Can you work these out from the drawing? Everything is in mm from the part's minimum corner. Coordinates: 2 decimals unless noted, no trailing zeros. Order: outer loops, then holes, each group sorted by start corner. A loop starts at its lowest first (then second) coordinate and runs counter-clockwise, first axis right, second up. Notation, with made-up numbers: (-23, 41) -> (-8, 41) arc R29 cw to (-8, 66) -> close; hole circle Ø7 at (61, -15). An arc over 180 degrees is marked (long way). Use a Markdown table: item, result. Add a question column.
1) Will these pins go through, and if not, where does the flat tip stop? pin 1 Ø2 at (x, y) = (44, 1) entering from -Z; pin 2 Ø2.5 at (y, z) = (2, 14.5) entering from +X.
2) If we section it at A-A (x = 28): Write out the boundary of the cut face in (y, z), plus the area to 4 significant figures.
3) If we section it at B-B (z = 70): Write out the boundary of the cut face in (x, y).
4) If we section it at D-D (y = 2.85): Give the number of separate pieces and of enclosed holes in the cut face, plus the area to 3 significant figures.
5) If I drill on L1, parallel to X at y = 2.8, z = 70; L2, parallel to Z at x = 36.5, y = 4.15; L3, parallel to Z at x = 28.5, y = 3.75, over which ranges is the centre line in solid material (lowest first)? Write a range as [from, to].
6) If we section it at C-C (x = 56): Write out the boundary of the cut face in (y, z).
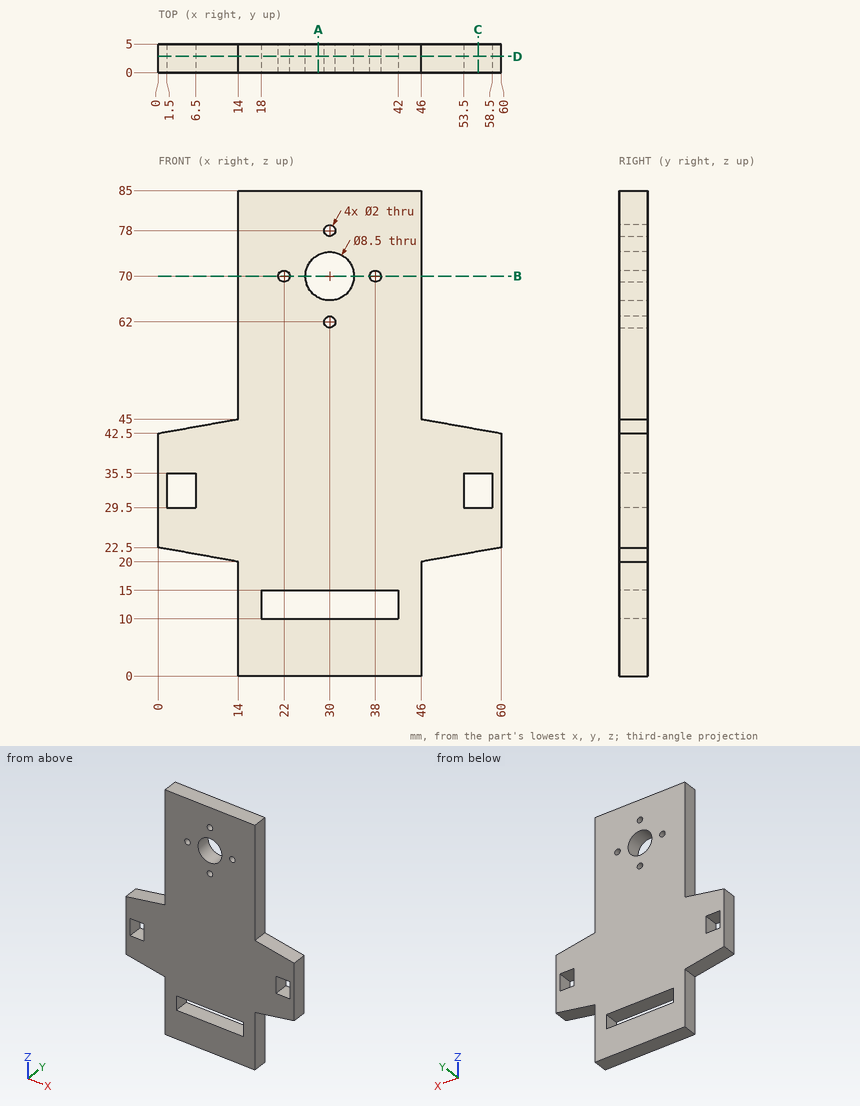
Answer sheet:
| question | item | result |
|---|---|---|
| 1 | pin 1 | z = 0 |
| 1 | pin 2 | x = 46 |
| 2 | outline | (0, 0) -> (5, 0) -> (5, 10) -> (0, 10) -> close; (0, 15) -> (5, 15) -> (5, 66.25) -> (0, 66.25) -> close; (0, 73.75) -> (5, 73.75) -> (5, 85) -> (0, 85) -> close |
| 2 | area | 362.5 mm2 |
| 3 | outline | (14, 0) -> (21, 0) -> (21, 5) -> (14, 5) -> close; (23, 0) -> (25.75, 0) -> (25.75, 5) -> (23, 5) -> close; (34.25, 0) -> (37, 0) -> (37, 5) -> (34.25, 5) -> close; (39, 0) -> (46, 0) -> (46, 5) -> (39, 5) -> close |
| 4 | separate pieces | 1 |
| 4 | enclosed holes | 8 |
| 4 | area | 3,100 mm2 |
| 5 | L1 | [14, 21], [23, 25.75], [34.25, 37], [39, 46] |
| 5 | L2 | [0, 10], [15, 85] |
| 5 | L3 | [0, 10], [15, 66.02], [73.98, 85] |
| 6 | outline | (0, 21.79) -> (5, 21.79) -> (5, 29.5) -> (0, 29.5) -> close; (0, 35.5) -> (5, 35.5) -> (5, 43.21) -> (0, 43.21) -> close |
